```python
from build123d import *

# Parameters (mm, degrees)
F0_W     = 90
F0_H     = 60
F1_DEPTH = 50
F2_R     = 7.5
F3_DEPTH = 25
F5_DEPTH = 50
F7_DEPTH = 95


with BuildPart() as f1:
    # F0 (on Top) → F1 (new body)
    with BuildSketch(Plane.XY):
        Rectangle(F0_W, F0_H)
    extrude(amount=F1_DEPTH)

    # F2 (on face) → F3 (join)
    with BuildSketch(Plane.XZ.offset(30)):
        with Locations((0, 20)):
            Circle(F2_R)
    extrude(amount=F3_DEPTH)

    # F4 (on face) → F5 (join)
    with BuildSketch(Plane.XY.offset(50)):
        Polygon((-14.433757, -25), (14.433757, -25), (28.867513, 0), (14.433757, 25), (-14.433757, 25), (-28.867513, 0), align=None)
    extrude(amount=F5_DEPTH)

    # F6 (on face) → F7 (cut)
    with BuildSketch(Plane.XY.offset(100)):
        Polygon((12.990381, 7.5), (0, 15), (-12.990381, 7.5), (-12.990381, -7.5), (0, -15), (12.990381, -7.5), align=None)
    extrude(amount=-F7_DEPTH, mode=Mode.SUBTRACT)


solid = f1.part
```
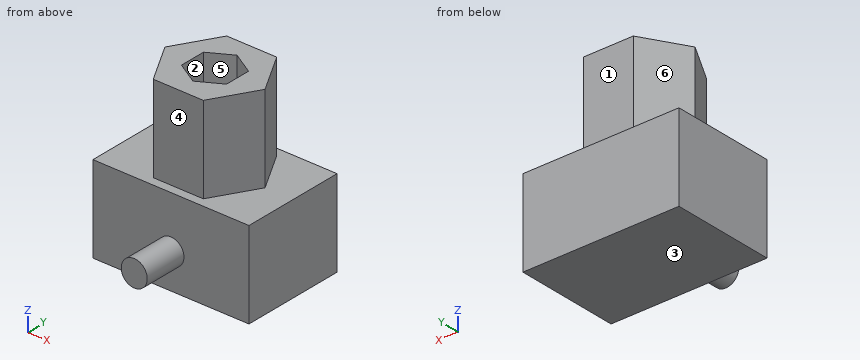
Part model, mm, in its own coordinate system. Face numbers are marked on the shaded views. A direction names the side the tool comes from. Coordinates: 2 decimals unless noted, no trailing zeros. Write each loop counter-clockwise with the first axis right and the second up, starting at its lowest first coordinate (ties: lowest second). Pieces come first, ordered by that corner, then holes.
Item 1: Pin check, flat tips, straight feed: pin 1 (8 mm diameter, centred on x = -4.5, y = -2, fed in from +Z); pin 2 (5 mm diameter, centred on x = 24, y = -29, fed in from +Z); pin 3 (1.5 mm diameter, centred on y = 0.5, z = 54, fed in from +X). Stop position of each tip, or through.
Item 2: Slice it at A-A (z = 84). Write the cut outline in (x, y), and give its area (3 significant figures).
Item 3: Mould opens along Y. For the marked faces 1, 2 and 3 say: released by +Y, released by -Y, zero draft, split by the parting line, or undercut.
Item 4: Slice it at B-B (x = 11.5). Write the cut outline in (y, z), and give its area (3 significant figures).
Item 5: Probe line 1 (X direction, y = -2, z = 15.5); line 2 (Y direction, x = 36, z = 20); line 3 (Y direction, x = 3.5, z = 56). List the from-to ranges inside material, lowest first.
Item 6: Slice it at C-C (y = 11). Write the cut outline in (x, z).
Item 7: Slice it at D-D (z = 20). Write the cut outline in (x, y).
Item 8: Which spindle directions (+Z, -Z, +X, -X, +Y, -Y) get a long thin tool onto all of the face, cutting with end or side? Do the marked faces 4, 5 and 6. Say none if no direction does.
Results found:
1. pin 1: stops at z = 5
1. pin 2: stops at z = 50
1. pin 3: stops at x = 28.87
2. outline: (-28.87, 0) - (-14.43, -25) - (14.43, -25) - (28.87, 0) - (14.43, 25) - (-14.43, 25) - close; hole (-12.99, -7.5) - (0, -15) - (12.99, -7.5) - (12.99, 7.5) - (0, 15) - (-12.99, 7.5) - close
2. area: 1,580 mm2
3. face 1: released by +Y
3. face 2: undercut
3. face 3: zero draft
4. outline: (-30, 0) - (30, 0) - (30, 50) - (25, 50) - (25, 100) - (8.36, 100) - (8.36, 5) - (-8.36, 5) - (-8.36, 100) - (-25, 100) - (-25, 50) - (-30, 50) - close
4. area: 3,910 mm2
5. line 1: x = -45 to -12.99, 12.99 to 45
5. line 2: y = -30 to 30
5. line 3: y = -25 to -12.98, 12.98 to 25
6. outline: (-45, 0) - (45, 0) - (45, 50) - (22.52, 50) - (22.52, 100) - (6.93, 100) - (6.93, 5) - (-6.93, 5) - (-6.93, 100) - (-22.52, 100) - (-22.52, 50) - (-45, 50) - close
7. outline: (-45, -30) - (-7.5, -30) - (-7.5, -55) - (7.5, -55) - (7.5, -30) - (45, -30) - (45, 30) - (-45, 30) - close; hole (-12.99, -7.5) - (0, -15) - (12.99, -7.5) - (12.99, 7.5) - (0, 15) - (-12.99, 7.5) - close
8. face 4: +Z, +X, -X, -Y
8. face 5: +Z
8. face 6: +Z, -X, +Y
